from build123d import *

# Parameters (mm, degrees)
F0_W      = 12
F0_H      = 12
F1_DEPTH  = 3.5
F2_R      = 0.5
F3_R      = 4
F4_DEPTH  = 0.75
F5_R      = 0.1
F6_R      = 0.1
F7_W      = 3.8
F7_H      = 1
F7_W_2    = 1.2
F8_DEPTH  = 0.3
F9_W      = 1.2
F9_H      = 1
F9_W_2    = 3.8
F10_DEPTH = 0.3
F12_DEPTH = 1.4


with BuildPart() as f1:
    # F0 (on Front) → F1 (new body)
    with BuildSketch(Plane.XZ):
        Rectangle(F0_W, F0_H)
    extrude(amount=F1_DEPTH)

    # F2
    f2_edges = [f1.edges().sort_by_distance(p)[0] for p in [
        (6, -1.75, 6),
        (6, -1.75, -6),
        (-6, -1.75, -6),
        (-6, -1.75, 6),
    ]]
    fillet(f2_edges, radius=F2_R)

    # F3 (on face) → F4 (join)
    with BuildSketch(Plane.XZ.offset(3.5)):
        Circle(F3_R)
    extrude(amount=F4_DEPTH)

    # F5
    f5_edges = [f1.edges().sort_by_distance(p)[0] for p in [
        (-4, -4.25, 0),
    ]]
    fillet(f5_edges, radius=F5_R)

    # F6
    f6_edges = [f1.edges().sort_by_distance(p)[0] for p in [
        (0, -3.5, -6),
        (-5.853553, -3.5, -5.853553),
        (5.853553, -3.5, -5.853553),
        (-6, -3.5, 0),
        (6, -3.5, 0),
        (-5.853553, -3.5, 5.853553),
        (5.853553, -3.5, 5.853553),
        (0, -3.5, 6),
        (-4, -3.5, 0),
    ]]
    fillet(f6_edges, radius=F6_R)

    # F7 (on face) → F8 (join)
    with BuildSketch(Plane(origin=(-6, 0, 0), x_dir=(0, -1, 0), z_dir=(-1, 0, 0))):
        with Locations((-1.9, 2.5)):
            Rectangle(F7_W, F7_H)
        with Locations((0.6, 2.5)):
            Rectangle(F7_W_2, F7_H)
        with Locations((0.6, -2.5)):
            Rectangle(F7_W_2, F7_H)
        with Locations((-1.9, -2.5)):
            Rectangle(F7_W, F7_H)
    extrude(amount=F8_DEPTH)

    # F9 (on face) → F10 (join)
    with BuildSketch(Plane.YZ.offset(6)):
        with Locations((-0.6, 2.5)):
            Rectangle(F9_W, F9_H)
        with Locations((1.9, 2.5)):
            Rectangle(F9_W_2, F9_H)
        with Locations((-0.6, -2.5)):
            Rectangle(F9_W, F9_H)
        with Locations((1.9, -2.5)):
            Rectangle(F9_W_2, F9_H)
    extrude(amount=F10_DEPTH)

    # F11 (on face) → F12 (join)
    with BuildSketch(Plane(origin=(0, 0, 0), x_dir=(-1, 0, 0), z_dir=(0, 1, 0))):
        with BuildLine():
            Line((0.9, 4.475), (-0.85, 4.475))
            ThreePointArc((-0.85, 4.475), (0.025, 3.6496433929), (0.9, 4.475))
        make_face()
        with BuildLine():
            Line((-0.85, -4.475), (0.9, -4.475))
            ThreePointArc((0.9, -4.475), (0.025, -3.6496433929), (-0.85, -4.475))
        make_face()
    extrude(amount=F12_DEPTH)


solid = f1.part
Geometry check sheet. Reference: the model listing, model coordinates, mm. A direction names the side the tool comes from. Round coordinates to 2 decimals unless told otherwise and drop trailing zeros. Loops run counter-clockwise (first coordinate to the right, second up) from the corner with the lowest first, then second, coordinate; pieces in that order, holes last. Notation, with made-up numbers: (63, 83) - (72, 83) arc R8 ccw to (72, 94) - close; hole circle Ø7 at (-9.5, 67.25). An arc over 180 degrees is marked (long way). One line per question, with ' | ' between items. Start each with the question number.
1. Scan lines: line 1 (Y direction, x = 4.75, z = 2.75); line 2 (X direction, y = -1.25, z = -1.5); line 3 (Y direction, x = 3.25, z = 1.75). Record each from-to range of solid material in increasing order. Write a range as [from, to].
2. Draft check along X on faces 5 (the face through (6.3, 1.3, -2.5)), 6 (the face through (0, 1.4, -4)), 7 (the face through (-6, 1.9, -2.5)). Enter one of: released by +X, released by -X, zero draft, split by the parting line, or undercut.
3. Cross-section at B-B on x = 0. Record the cut outline in (y, z) (3 decimals), then the cut area to 3 significant figures.
4. Depth check by flat-ended pin: pin 1 (3.5 mm diameter, centred on x = -0.5, z = 1.5, fed in from +Y); pin 2 (0.7 mm diameter, centred on x = -0.5, y = 1, fed in from +Z) (3 decimals); pin 3 (1.5 mm diameter, centred on x = 4.5, z = 4.5, fed in from -Y). Enter the tip coordinate at first touch or a pass-through.
5. Cross-section at C-C on z = 0. Record the cut outline in (x, y).
6. Tool access check on faces 1 (the face through (6, 1.9, 2.5)), 2 (the face through (0, 1.4, 4)), 3 (the face through (-0.04, 0.69, -3.65)), 4 (the face through (0, 1, 4.475)). Record the directions out of +Z, -Z, +X, -X, +Y, -Y that give a thin tool (end or side, any length) a straight path to the whole face; none if there is none.
7. Cross-section at D-D on y = 2.75. Record the cut outline in (x, z).
8. Cross-section at A-A on y = 0.75. State how many separate pieces and enclosed holes the cut face has, then the cut area to 3 significant figures.
Taken from the geometry:
1) line 1: [-3.5, 0] | line 2: [-6, 6] | line 3: [-4.25, 0]
2) face 5: released by +X | face 6: zero draft | face 7: undercut
3) outline: (-4.25, -3.9) arc R0.1 ccw to (-4.15, -4) - (-3.6, -4) arc R0.1 cw to (-3.5, -4.1) - (-3.5, -5.9) arc R0.1 ccw to (-3.4, -6) - (0, -6) - (0, -4.475) - (1.4, -4.475) - (1.4, -3.65) - (0, -3.65) - (0, 3.65) - (1.4, 3.65) - (1.4, 4.475) - (0, 4.475) - (0, 6) - (-3.4, 6) arc R0.1 ccw to (-3.5, 5.9) - (-3.5, 4.1) arc R0.1 cw to (-3.6, 4) - (-4.15, 4) arc R0.1 ccw to (-4.25, 3.9) - close | area: 50.3 mm²
4) pin 1: y = 0 | pin 2: z = 4.475 | pin 3: y = -3.5
5) outline: (-6, -3.4) arc R0.1 ccw to (-5.9, -3.5) - (-4.1, -3.5) arc R0.1 cw to (-4, -3.6) - (-4, -4.15) arc R0.1 ccw to (-3.9, -4.25) - (3.9, -4.25) arc R0.1 ccw to (4, -4.15) - (4, -3.6) arc R0.1 cw to (4.1, -3.5) - (5.9, -3.5) arc R0.1 ccw to (6, -3.4) - (6, 0) - (-6, 0) - close
6) face 1: +Z, -Z, +Y | face 2: +Z, -Z, +X, -X, +Y | face 3: +Y | face 4: +Z, +X, -X, +Y
7) outline: (-6.3, -3) - (-6, -3) - (-6, -2) - (-6.3, -2) - close; (-6.3, 2) - (-6, 2) - (-6, 3) - (-6.3, 3) - close; (6, -3) - (6.3, -3) - (6.3, -2) - (6, -2) - close; (6, 2) - (6.3, 2) - (6.3, 3) - (6, 3) - close
8) separate pieces: 6 | enclosed holes: 0 | area: 3.43 mm²
